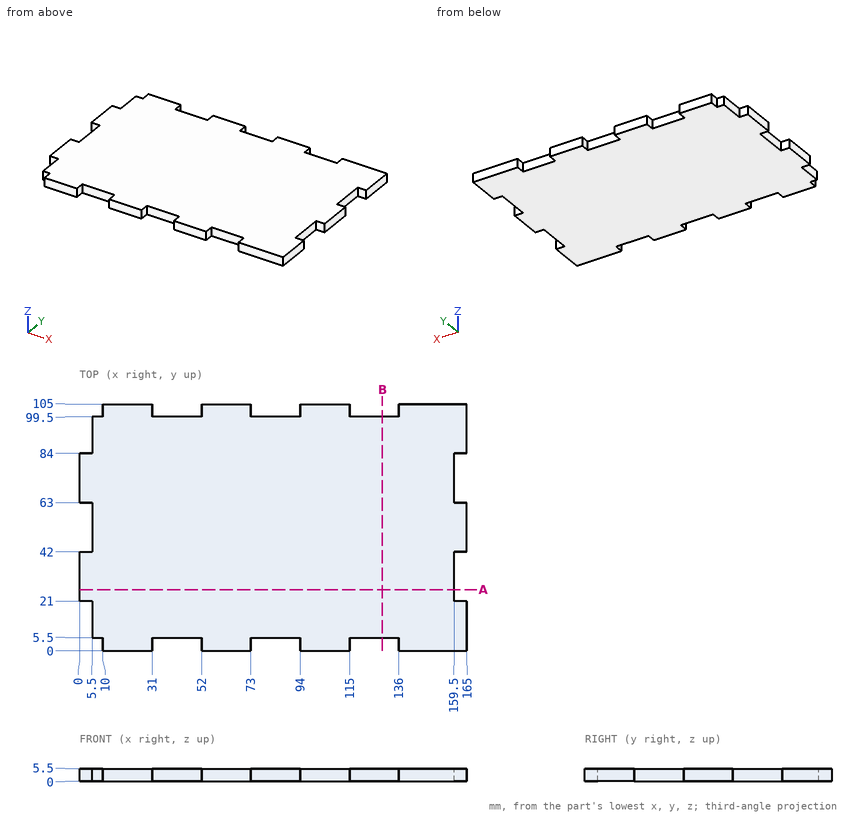
Job drawing, mm, ordinate dimensions from the low corner. One solid piece. Round coordinates to 2 decimals unless told otherwise and drop trailing zeros. Write each loop counter-clockwise with the first axis right and the second up, starting at its lowest first coordinate (ties: lowest second). Pieces come first, ordered by that corner, then holes.
1) Pin check, flat tips, straight feed: pin 1 (3 mm diameter, centred on y = 88.5, z = 2.5, fed in from -X); pin 2 (3 mm diameter, centred on x = 45, z = 3, fed in from +Y); pin 3 (3 mm diameter, centred on y = 1.5, z = 2.5, fed in from -X). Stop position of each tip, or through.
2) Drill centre lines: probe 1 along X at (y, z) = (8.5, 3.7); probe 2 along X at (y, z) = (76.5, 2.9); probe 3 along Y at (x, z) = (121.5, 3.05). Where is each one in solid material? Low to high.
3) Band-saw the part on A-A, the plane y = 26. List the corners of the cut face in (x, z), and give its area (3 significant figures).
4) Band-saw the part on B-B, the plane x = 129. List the corners of the cut face in (y, z), and give its area (3 significant figures).
Ans:
1. pin 1: stops at x = 5.5
1. pin 2: stops at y = 99.5
1. pin 3: stops at x = 10
2. probe 1: x = 5.5 to 165
2. probe 2: x = 0 to 159.5
2. probe 3: y = 5.5 to 99.5
3. outline: (0, 0) - (159.5, 0) - (159.5, 5.5) - (0, 5.5) - close
3. area: 877 mm2
4. outline: (5.5, 0) - (99.5, 0) - (99.5, 5.5) - (5.5, 5.5) - close
4. area: 517 mm2
